from build123d import *

# Parameters (mm, degrees)
MAINBASESKETCH_W             = 15.8
MAINBASESKETCH_H             = 3.2
MAINBASEEXTRUDE_DEPTH        = 7.9
STUDSSKETCH_R                = 2.4
STUDSEXTRUDE_DEPTH           = 1.6
STUDSPATTERN_COUNT           = 2
STUDSPATTERN_PITCH           = 8
STUDSPATTERN_COUNT_DIR2      = 2
STUDSPATTERN_PITCH_DIR2      = 8
MAINBASESHELL_T              = -1.2
LCUTBLUE_DEPTH               = 19.555463972
LCUTBLUE_DEPTH_BACK          = 19.555463972
CUTADDEDTOLCUT_DEPTH         = 2
MADESLIMCUTSKETCH_W          = 7.9
MADESLIMCUTSKETCH_H          = 7.9
MADESLIMCUT_DEPTH            = 19.897228453
MADESLIMFILLEXT_REACH        = 20.897
SKETCH33_W                   = 5.500952983
SKETCH33_H                   = 1.199047018
SHORTLEXTENSIONSKETCH_W      = 1.583745828
SHORTLEXTENSIONSKETCH_H      = 7.9
SHORTLEXTENDEDCUTSKETCH_W    = 13.4
SHORTLEXTENDEDCUTSKETCH_H    = 1.582792846
SHORTLEXTENDEDCUT_DEPTH      = 2
SHORTLUNDERSTUMPS_START      = -0.2
SHORTLUNDERSTUMPSKETCH_W     = 0.996828098
SHORTLUNDERSTUMPSKETCH_H     = 1
SHORTLUNDERSTUMPS_DEPTH      = 1.6
SHORTLUPPERCIRCLES_START     = -0.2
SHORTLUPPERCIRCLESSKETCH_R   = 2.25
SHORTLUPPERCIRCLESSKETCH_R_2 = 2
SHORTLUPPERCIRCLES_DEPTH     = 1.5
CUT_EXTRUDE17_DEPTH          = 7.9
SKETCH60_W                   = 1.205928798
SKETCH60_H                   = 7.083745828
SKETCH63_W                   = 1.583745828
SKETCH63_H                   = 7.9
LPATTERN2_START              = -2.883745828
LPATTERN2_OUTLINE_R          = 2.25
LPATTERN2_OUTLINE_R_2        = 2
LPATTERN2_DEPTH              = 1.3
FILLET4_R                    = 1
FILLET16_R                   = 2


# Read off the part's stored shape, not the designer's step: LPattern2
with BuildPart() as part:
    # MainBaseSketch → MainBaseExtrude (new, symmetric)
    with BuildSketch(Plane.XY):
        with Locations((8.581967213, 1.6)):
            Rectangle(MAINBASESKETCH_W, MAINBASESKETCH_H)
    extrude(amount=MAINBASEEXTRUDE_DEPTH, both=True)

    # StudsSketch → StudsExtrude (add)
    with BuildSketch(Plane(origin=(0, 3.2, 0), x_dir=(1, 0, 0), z_dir=(0, 1, 0))):
        with Locations((4.581967213, 4)):
            Circle(STUDSSKETCH_R)
    studsextrude = extrude(amount=STUDSEXTRUDE_DEPTH)

    # StudsPattern: StudsExtrude 2 × 2
    with Locations(*[(j * STUDSPATTERN_PITCH_DIR2, 0, i * STUDSPATTERN_PITCH) for i in range(STUDSPATTERN_COUNT) for j in range(STUDSPATTERN_COUNT_DIR2) if (i, j) != (0, 0)]):
        add(studsextrude)

    # MainBaseShell
    mainbaseshell_openings = [part.faces().sort_by_distance(p)[0] for p in [
        (8.581967213, 0, 0),
    ]]
    offset(amount=MAINBASESHELL_T, openings=mainbaseshell_openings, kind=Kind.INTERSECTION)

    # LCUTBlueSketch → LCutBlue (cut, two sides: drawn at the far end of the back side and taken through both)
    with BuildSketch(Plane(origin=(0, 3.2, 0), x_dir=(1, 0, 0), z_dir=(0, 1, 0)).offset(-LCUTBLUE_DEPTH_BACK)):
        Polygon((8.581967213, 53.229874044), (8.581967213, 7.9), (8.581967213, 0), (16.481967213, 0), (61.811841258, 0), (125.917963912, 64.106122654), (72.688089868, 117.335996699), align=None)
    extrude(amount=LCUTBLUE_DEPTH + LCUTBLUE_DEPTH_BACK, mode=Mode.SUBTRACT)

    # CutAddedtoLSketch → CutAddedToLCut (add)
    with BuildSketch(Plane.XZ):
        Polygon((7.382920196, -6.7), (8.581967213, -6.7), (8.581967213, 0), (15.281967213, 0), (15.281967213, 1.199047018), (7.382920196, 1.199047018), (7.382920196, 0), align=None)
    extrude(amount=-CUTADDEDTOLCUT_DEPTH)

    # MadeSlimCutSketch → MadeSlimCut (cut, through all)
    with BuildSketch(Plane.XZ):
        with Locations((4.631967213, -3.95)):
            Rectangle(MADESLIMCUTSKETCH_W, MADESLIMCUTSKETCH_H)
    extrude(amount=-MADESLIMCUT_DEPTH, mode=Mode.SUBTRACT)

    # Sketch33 → MadeSlimFillExt (add, up to next)
    with BuildSketch(Plane.XZ, mode=Mode.PRIVATE) as madeslimfillext_sk1:
        with Locations((4.632443704, 0.599523509)):
            Rectangle(SKETCH33_W, SKETCH33_H)
    madeslimfillext_tool1 = extrude(madeslimfillext_sk1.sketch, amount=-MADESLIMFILLEXT_REACH, mode=Mode.PRIVATE) - part.part
    add(madeslimfillext_tool1.solids().sort_by_distance((4.632444, 0, 0.599524))[0])

    # ShortLExtension: sweep along a curve in space
    with BuildLine() as shortlextension_path:
        Line((0.681967213, 3.2, 0), (16.481967213, 3.2, 0))
    # ShortLExtensionSketch → ShortLExtension (sweep)
    with BuildSketch(Plane(origin=(16.481967213, 0, 0), x_dir=(0, 0, -1), z_dir=(1, 0, 0))):
        with Locations((0.791872914, 3.95)):
            Rectangle(SHORTLEXTENSIONSKETCH_W, SHORTLEXTENSIONSKETCH_H)
    sweep(path=shortlextension_path.line)

    # ShortLExtendedCutSketch → ShortLExtendedCut (cut)
    with BuildSketch(Plane.XZ):
        with Locations((8.581967213, 0.407650595)):
            Rectangle(SHORTLEXTENDEDCUTSKETCH_W, SHORTLEXTENDEDCUTSKETCH_H)
    extrude(amount=-SHORTLEXTENDEDCUT_DEPTH, mode=Mode.SUBTRACT)

    # ShortLUnderStumpSketch → ShortLUnderStumps (add)
    with BuildSketch(Plane.XZ.offset(-2).offset(SHORTLUNDERSTUMPS_START)):
        with Locations((4.581764801, 0.116254172)):
            Rectangle(SHORTLUNDERSTUMPSKETCH_W, SHORTLUNDERSTUMPSKETCH_H)
        with Locations((8.57767054, 0.116254172)):
            Rectangle(SHORTLUNDERSTUMPSKETCH_W, SHORTLUNDERSTUMPSKETCH_H)
        with Locations((12.582169625, 0.116254172)):
            Rectangle(SHORTLUNDERSTUMPSKETCH_W, SHORTLUNDERSTUMPSKETCH_H)
    extrude(amount=SHORTLUNDERSTUMPS_DEPTH)

    # ShortLUpperCirclesSketch → ShortLUpperCircles (add)
    # profile 1 of 2: a face of its own
    with BuildSketch(Plane(origin=(0, 0, -1.583745828), x_dir=(-1, 0, 0), z_dir=(0, 0, -1)).offset(SHORTLUPPERCIRCLES_START)):
        with Locations(Location((-12.581967213, 3.95, 0), (0, 0, 90))):
            Circle(SHORTLUPPERCIRCLESSKETCH_R)
        with Locations(Location((-12.581967213, 3.95, 0), (0, 0, 90))):
            Circle(SHORTLUPPERCIRCLESSKETCH_R_2, mode=Mode.SUBTRACT)
    # profile 2 of 2: a face of its own
    with BuildSketch(Plane(origin=(0, 0, -1.583745828), x_dir=(-1, 0, 0), z_dir=(0, 0, -1)).offset(SHORTLUPPERCIRCLES_START)):
        with Locations(Location((-4.581967213, 3.95, 0), (0, 0, 270))):
            Circle(SHORTLUPPERCIRCLESSKETCH_R)
        with Locations(Location((-4.581967213, 3.95, 0), (0, 0, 270))):
            Circle(SHORTLUPPERCIRCLESSKETCH_R_2, mode=Mode.SUBTRACT)
    extrude(amount=SHORTLUPPERCIRCLES_DEPTH)

    # Sketch59 → Cut-Extrude17 (cut)
    with BuildSketch(Plane.ZY.offset(-8.581967213)):
        Polygon((-1.583745828, 6.2), (-1.583745828, 7.9), (0, 7.9), (0, 3.2), (1.6, 3.2), (1.6, 4.8), (6.4, 4.8), (6.4, 3.2), (7.9, 3.2), (7.9, 0), (-1.583745828, 0), (-1.583745828, 1.7), (-2.883745828, 1.7), (-2.883745828, 6.2), align=None)
    extrude(amount=-CUT_EXTRUDE17_DEPTH, mode=Mode.SUBTRACT)

    # Sweep4: sweep along a curve in space
    with BuildLine() as sweep4_path:
        Line((8.581967213, 0, 6.7), (8.581967213, 2, 6.7))
    # Sketch60 → Sweep4 (sweep)
    with BuildSketch(Plane(origin=(0, 0, 0), x_dir=(-1, 0, 0), z_dir=(0, -1, 0))):
        with Locations((-7.979002814, -3.158127086)):
            Rectangle(SKETCH60_W, SKETCH60_H)
    sweep(path=sweep4_path.line)

    # Sweep5: sweep along a curve in space
    with BuildLine() as sweep5_path:
        Line((0.681967213, 7.9, 0), (8.581967213, 7.9, 0))
    # Sketch63 → Sweep5 (sweep)
    with BuildSketch(Plane.ZY.offset(-0.681967213)):
        with Locations((-0.791872914, 11.85)):
            Rectangle(SKETCH63_W, SKETCH63_H)
    sweep(path=sweep5_path.line)

    # LPattern2 outline → LPattern2 (add)
    with BuildSketch(Plane.XY.offset(LPATTERN2_START)):
        with Locations((4.581967213, 11.95)):
            Circle(LPATTERN2_OUTLINE_R)
        with Locations((4.581967213, 11.95)):
            Circle(LPATTERN2_OUTLINE_R_2, mode=Mode.SUBTRACT)
    extrude(amount=LPATTERN2_DEPTH)

    # Fillet4
    fillet4_edges = [part.edges().sort_by_distance(p)[0] for p in [
        (0.681967213, 15.8, -0.791872914),
        (8.581967213, 15.8, -0.791872914),
    ]]
    fillet(fillet4_edges, radius=FILLET4_R)

    # Fillet16
    fillet16_edges = [part.edges().sort_by_distance(p)[0] for p in [
        (8.581967213, 1.6, 7.9),
        (0.681967213, 1.6, 7.9),
    ]]
    fillet(fillet16_edges, radius=FILLET16_R)


solid = part.part
Model file for the job. Use its own axes, mm. A direction names the side the tool comes from. Round coordinates to 2 decimals unless told otherwise and drop trailing zeros. Loops run counter-clockwise (first coordinate to the right, second up) from the corner with the lowest first, then second, coordinate; pieces in that order, holes last.
1. Mould opens along Z. For faces 1 (the flat face through (5, 12, -1.584)), 2 (the cylindrical face through (5.69, 2.79, 4.46)), 3 (the flat face through (5, 2, 7.9)), 4 (the cylindrical face through (0.98, 15.51, -0.8)) say: +Z half, -Z half, draft (parallel to the pull), parting line (faces both ways), or undercut.
Check values:
face 1: -Z half
face 2: undercut
face 3: +Z half
face 4: draft
2. Wall check: probe 1 along X at (y, z) = (3.95, -2.5); probe 2 along Z at (x, y) = (2, 15); probe 3 along Z at (x, y) = (4.75, 1.25). Give the ranges that are in metal, low to high.
Check values:
probe 1: x = 2.33 to 2.58, 6.58 to 6.83
probe 2: z = -1.58 to 0
probe 3: z = -1.58 to 0.62, 6.7 to 7.9
3. Tool access for faces 5 (the flat face through (5, 4.8, 4)), 6 (the flat face through (5, 4, -1.584)), 7 (the flat face through (3, 3.2, 2)): list every direction of +Z, -Z, +X, -X, +Y, -Y with a clear straight run to the whole face (end or side of a thin tool).
Check values:
face 5: +Z, +X, -X, +Y
face 6: -Z
face 7: +Y
4. Drop flat-ended pins along their axis: P1, Ø4.5, axis at x = 4.5, y = 12, coming from the -Z side; P2, Ø3, axis at x = 4.58, z = 4, coming from the -Y side; P3, Ø2, axis at x = 2, z = 2, coming from the +Y side; P4, Ø4.5, axis at x = 5, z = 2, coming from the -Y side. Give the stop position or say it passes through.
Check values:
P1: stops at z = -2.88
P2: stops at y = 2
P3: stops at y = 4.8
P4: stops at y = 0.6
5. Band-saw the part on A-A, the plane y = 3.95. List the corners of the cut face in (x, z), and give its area (3 significant figures).
Check values:
outline: (0.68, -1.58) - (2.33, -1.58) - (2.33, -2.88) - (2.58, -2.88) - (2.58, -1.58) - (6.58, -1.58) - (6.58, -2.88) - (6.83, -2.88) - (6.83, -1.58) - (8.58, -1.58) - (8.58, 0) - (0.68, 0) - close; circle Ø4.8 at (4.58, 4)
area: 31.3 mm2
6. Band-saw the part on C-C, the plane y = 11.95. List the corners of the cut face in (x, z).
Check values:
outline: (0.68, -1.58) - (2.33, -1.58) - (2.33, -2.88) - (2.58, -2.88) - (2.58, -1.58) - (6.58, -1.58) - (6.58, -2.88) - (6.83, -2.88) - (6.83, -1.58) - (8.58, -1.58) - (8.58, 0) - (0.68, 0) - close
7. Band-saw the part on D-D, the plane z = -2. List the corners of the cut face in (x, y), and give its area (3 significant figures).
Check values:
outline: circle Ø4.5 at (4.58, 3.95); circle Ø4.5 at (4.58, 11.95); hole circle Ø4 at (4.58, 3.95); hole circle Ø4 at (4.58, 11.95)
area: 6.68 mm2
8. Band-saw the part on B-B, the plane z = 4. List the corners of the cut face in (x, y), and give its area (3 significant figures).
Check values:
outline: (0.68, 0) - (1.88, 0) - (1.88, 2) - (3.38, 2) - (3.38, 3.6) - (5.78, 3.6) - (5.78, 2) - (7.38, 2) - (7.38, 0) - (8.58, 0) - (8.58, 3.2) - (6.98, 3.2) - (6.98, 4.8) - (2.18, 4.8) - (2.18, 3.2) - (0.68, 3.2) - close
area: 18.1 mm2
